```python
from build123d import *

# Parameters (mm, degrees)
F4_R = 0.99999
F3_T = -0.5


# Not quite as in the source:
# - a fillet or chamfer is up to 0.001 mm smaller than in the source, because OpenCascade refuses the exact size


with BuildPart() as f2:
    # F0 (on Front) → F2 (revolve)
    with BuildSketch(Plane.XZ):
        Polygon((0, 4), (0, 0), (11, 0), (11.0396612436, 2.5), (2, 2.5), (2, 4), align=None)
    revolve(axis=Axis((6.7295320332, 0, 0), (1, 0, 0)))

    # F4 (radius 1 in the source; OpenCascade refuses exactly that, so slightly less here)
    f4_edges = [f2.edges().sort_by_distance(p)[0] for p in [
        (2, 0, -4),
        (0, 0, -4),
    ]]
    fillet(f4_edges, radius=F4_R)

    # F3
    f3_openings = [f2.faces().sort_by_distance(p)[0] for p in [
        (11.019831, 0, -1.25),
    ]]
    offset(amount=F3_T, openings=f3_openings, kind=Kind.INTERSECTION)


solid = f2.part
```
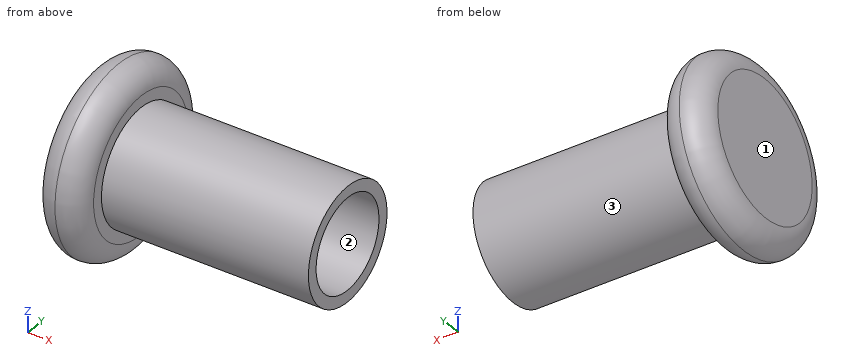
Verification items for the finished model (mm, model axes). Face numbers are marked on the shaded views. Coordinates: 2 decimals unless noted, no trailing zeros. Order: outer loops, then holes, each group sorted by start corner. A loop starts at its lowest first (then second) coordinate and runs counter-clockwise, first axis right, second up. Notation, with made-up numbers: (-9, 18.25) -> (38, 18.25) arc R10 cw to (38, 24.25) -> close; hole circle Ø8 at (32, -30.75). An arc over 180 degrees is marked (long way). Answer as CSV lines item,"result". Start each with the question number.
1) Gauge pin test, flat ends, axial feed: pin 1 Ø2 at (x, y) = (6, 1) entering from -Z; pin 2 Ø1.5 at (x, z) = (2.5, 1.5) entering from +Y; pin 3 Ø4 at (x, z) = (7.5, -1.5) entering from -Y. Record the tip position at first contact, or that the pin passes through.
2) Release check for a two-part mould opening along Y. For the marked faces 1, 2 and 3 record: released by +Y, released by -Y, zero draft, split by the parting line, or undercut.
3) Cross-section at C-C, the plane x = 9. Record the boundary of the cut face in (y, z).
4) Material ranges on L1, parallel to Z at x = 8.75, y = 0; L2, parallel to Z at x = 1.05, y = 0; L3, parallel to X at y = -3, z = 0.25, recorded low to high. Write a range as [from, to].
Conclusion:
1,pin 1,"stops at z = -2.5"
1,pin 2,"stops at y = 3.39"
1,pin 3,"stops at y = -2.5"
2,face 1,"zero draft"
2,face 2,"undercut"
2,face 3,"split by the parting line"
3,outline,"circle Ø5 at (0, 0); hole circle Ø4 at (0, 0)"
4,L1,"z = [-2.5, -2], [2, 2.5]"
4,L2,"z = [-4, -3.5], [3.5, 4]"
4,L3,"x = [0, 0.5], [1.5, 2]"
